Autodesk Inventor part; units mm, degrees
ref_plane "YZ Plane" through (0, 0, 0) normal (1, 0, 0) x (0, 1, 0)
ref_plane "XZ Plane" through (0, 0, 0) normal (0, 1, 0) x (-1, 0, 0)
ref_plane "XY Plane" through (0, 0, 0) normal (0, 0, 1) x (1, 0, 0)
sketch "Sketch8" plane through (0, 0, 0) normal (0, 1, 0) x (-1, 0, 0)
  line L0 (-13.5, -17.5) -> (13.5, -17.5)
  line L1 (13.5, -17.5) -> (13.5, 17.5)
  line L2 (13.5, 17.5) -> (-13.5, 17.5)
  line L3 (-13.5, 17.5) -> (-13.5, -17.5)
  line L4 (-13.5, -17.5) -> (13.5, 17.5) construction
  line L5 (13.5, -17.5) -> (-13.5, 17.5) construction
  circle A0 centre (10, -7.5) radius 1.6
  circle A1 centre (10, 7.5) radius 1.6
  circle A2 centre (-10, 7.5) radius 1.6
  circle A3 centre (-10, -7.5) radius 1.6
  point P0 (0, 0)
  dimension "d38" = 35
  dimension "d39" = 27
  dimension "d40" = 20
  dimension "d41" = 15
  dimension "d42" = 7.5
  dimension "d43" = 10
  dimension "d44" = 3.2
extrude "Extrusion7" add sketch "Sketch8" against normal blind 3
sketch "Sketch14" plane through (0, 0, 0) normal (0, 1, 0) x (1, 0, 0)
  line L0 (-13.5, 17.5) -> (-13.5, -17.5)
  line L1 (-13.5, -17.5) -> (13.5, -17.5)
  line L2 (13.5, -17.5) -> (13.5, 17.5)
  line L3 (13.5, 17.5) -> (-13.5, 17.5)
  circle A0 centre (-10, 7.5) radius 1.6
  circle A1 centre (-10, -7.5) radius 1.6
  circle A2 centre (10, -7.5) radius 1.6
  circle A3 centre (10, 7.5) radius 1.6
  line L4 (13.5, -17.5) -> (13.5, 17.5)
  line L5 (13.5, 4.5) -> (7.5, 4.5)
  line L6 (7.5, 4.5) -> (7.5, -4.5)
  line L7 (7.5, -4.5) -> (13.5, -4.5)
  line L8 (13.5, -4.5) -> (13.5, 4.5)
  point P0 (0, 0)
  dimension "d79" = 7.5
  dimension "d80" = 3
  dimension "d81" = 3
extrude "Extrusion12" add sketch "Sketch14" along normal blind 22.3 contours L2 L7 L6 L5
sketch "Sketch15" plane through (13.5, -3, 17.5) normal (1, 0, 0) x (0, 0, -1)
  line L0 (0, 3) -> (13, 3)
  line L1 (0, 3) -> (0, 0)
  line L2 (35, 0) -> (0, 0)
  line L3 (35, 3) -> (35, 0)
  line L4 (22, 3) -> (35, 3)
  line L5 (22, 3) -> (22, 25.3)
  line L6 (13, 25.3) -> (22, 25.3)
  line L7 (13, 3) -> (13, 25.3)
  line L8 (35, 3) -> (35, 0)
  line L9 (35, 0) -> (41.8017, 14.6399)
  circle A0 centre (35, 17.8) radius 2.6
  circle A1 centre (35, 17.8) radius 7.5
  circle A2 centre (0, 17.8) radius 2.6
  circle A3 centre (0, 17.8) radius 7.5
  line L10 (-275, -9) -> (225, -9)
  line L11 (0, 0) -> (-6.8017, 14.6399)
  line L12 (0, 25.3) -> (35, 25.3)
  point P0 (17.5, 3)
  point P1 (13, 25.3)
  point P2 (22, 25.3)
  dimension "d84" = 5.2
  dimension "d85" = 35
  dimension "d86" = 17.5
  dimension "d87" = 26.8
  dimension "d88" = 15
extrude "Extrusion13" add sketch "Sketch15" against normal blind 3 contours L1 L11 A3 L12 L7 L0 | L3 L4 L5 L12 A1 L9 | A3 | A1
sketch "Sketch16" plane through (10.5, -3, 17.5) normal (-1, 0, 0) x (0, 0, 1)
  arc A0 (-35, 25.3) -> (-41.8017, 14.6399) centre (-35, 17.8) ccw
  line L0 (-41.8017, 14.6399) -> (-35, 0)
  line L1 (-35, 3) -> (-35, 0)
  line L2 (-26.5199, 3) -> (-35, 3)
  line L3 (-26.5199, 3) -> (-23.4801, 3)
  line L4 (-22, 3) -> (-23.4801, 3)
  line L5 (-22, 25.3) -> (-22, 3)
  line L6 (-22, 25.3) -> (-35, 25.3)
  circle A1 centre (-35, 17.8) radius 2.6
  arc A2 (6.8017, 14.6399) -> (0, 25.3) centre (0, 17.8) ccw
  line L7 (0, 25.3) -> (-13, 25.3)
  line L8 (-13, 3) -> (-13, 25.3)
  line L9 (-11.5199, 3) -> (-13, 3)
  line L10 (-11.5199, 3) -> (-8.4801, 3)
  line L11 (0, 3) -> (-8.4801, 3)
  line L12 (0, 0) -> (0, 3)
  line L13 (0, 0) -> (6.8017, 14.6399)
  circle A3 centre (0, 17.8) radius 2.6
  line L14 (-22, 3) -> (-29, 3)
  line L15 (-29, 3) -> (-29, 13)
  line L16 (-29, 13) -> (-22, 13)
  line L17 (-22, 13) -> (-22, 3)
  line L18 (-11.5199, 3) -> (-13, 3)
  line L19 (-13, 3) -> (-6, 3)
  line L20 (-6, 3) -> (-6, 13)
  line L21 (-6, 13) -> (-13, 13)
  line L22 (-13, 13) -> (-13, 3)
  line L23 (-23.4, 0) -> (-26.6, 0)
  line L24 (-26.6, 3) -> (-23.4, 3)
  line L25 (-8.4, 0) -> (-11.6, 0)
  line L26 (-11.6, 3) -> (-8.4, 3)
  point P0 (-17.5, 3)
  point P1 (-10, 0)
  point P2 (-6, 3)
  dimension "d91" = 7
  dimension "d92" = 3
  dimension "d93" = 10
extrude "Extrusion14" cut sketch "Sketch16" against normal blind 22.3 contours L5 L4 L3 L2 L15 L16 | L21 L20 L11 L10 L9 L8
sketch "Sketch17" plane through (10.5, -3, 17.5) normal (-1, 0, 0) x (0, 0, 1)
  circle A0 centre (-35, 17.8) radius 2.6
  line L0 (-29, 3) -> (-29, 13)
  line L1 (-29, 13) -> (-22, 13)
  line L2 (-22, 25.3) -> (-22, 13)
  line L3 (-22, 25.3) -> (-35, 25.3)
  arc A1 (-35, 25.3) -> (-41.8017, 14.6399) centre (-35, 17.8) ccw
  line L4 (-41.8017, 14.6399) -> (-35, 0)
  line L5 (-35, 3) -> (-35, 0)
  line L6 (-29, 3) -> (-35, 3)
  circle A2 centre (0, 17.8) radius 2.6
  line L7 (-13, 13) -> (-6, 13)
  line L8 (-6, 13) -> (-6, 3)
  line L9 (0, 3) -> (-6, 3)
  line L10 (0, 0) -> (0, 3)
  line L11 (0, 0) -> (6.8017, 14.6399)
  arc A3 (6.8017, 14.6399) -> (0, 25.3) centre (0, 17.8) ccw
  line L12 (0, 25.3) -> (-13, 25.3)
  line L13 (-13, 13) -> (-13, 25.3)
  line L14 (-13, 13) -> (-10, 25.3)
  line L15 (-22, 13) -> (-25, 25.3)
  line L16 (-35, 25.3) -> (0, 25.3)
  point P0 (-17.5, 3)
  dimension "d96" = 15
extrude "Extrusion15" add sketch "Sketch17" along normal up to surface (3 mm away) contours L12 L14 L13 | L15 L3 L2
fillet "Fillet2" radius 2 2 edges at (9, 22.3, -7.5) (9, 22.3, 7.5)
mirror "Mirror1" about plane through (0, 0, 0) normal (1, 0, 0) of "Extrusion12", "Extrusion13", "Extrusion14", "Extrusion15", "Fillet2"
chamfer "Chamfer1" distance 5 angle 45 4 edges at (-10.5, 0, 14.5) (-10.5, 0, -14.5) (10.5, 0, 14.5) (10.5, 0, -14.5)
sketch "Sketch18" plane through (-13.5, 22.3, -17.5) normal (-1, 0, 0) x (0, 0, 1)
  line L0 (13, -22.3) -> (6, -22.3)
  line L1 (6, -22.3) -> (6, -12.3)
  line L2 (6, -12.3) -> (13, -12.3)
  line L3 (13, -12.3) -> (13, -22.3)
  line L4 (29, -22.3) -> (22, -22.3)
  line L5 (22, -22.3) -> (22, -12.3)
  line L6 (22, -12.3) -> (29, -12.3)
  line L7 (29, -12.3) -> (29, -22.3)
  circle A0 centre (0, -7.5) radius 2.6
  circle A1 centre (35, -7.5) radius 2.6
  line L8 (41.8017, -10.6601) -> (35, -25.3)
  arc A2 (41.8017, -10.6601) -> (35, 0) centre (35, -7.5) ccw
  line L9 (0, 0) -> (35, 0)
  arc A3 (0, 0) -> (-6.8017, -10.6601) centre (0, -7.5) ccw
  line L10 (0, -25.3) -> (-6.8017, -10.6601)
  line L11 (35, -25.3) -> (0, -25.3)
  point P0 (17.5, -22.3)
  point P1 (17.5, -7)
  point P2 (17.5, -15.3)
  dimension "d103" = 7
  dimension "d104" = 10
hole "Hole3" at (-13.5, 15.3, 0) at (-13.5, 7, 0) direction (1, 0, 0) diameter 3.6 end through all
sketch "Sketch19" plane through (13.5, 22.3, 17.5) normal (1, 0, 0) x (0, 0, -1)
  circle A0 centre (17.5, -15.3) radius 1.8
  circle A1 centre (17.5, -7) radius 1.8
  circle A2 centre (17.5, -15.3) radius 3.25
  circle A3 centre (17.5, -7) radius 3.25
  point P0 (17.5, -22.3)
  dimension "d112" = 6.5
extrude "Extrusion16" cut sketch "Sketch19" against normal blind 3 contours A0 | A1 | A2 | A3
sketch "Sketch20" plane through (-13.5, 22.3, -17.5) normal (-1, 0, 0) x (0, 0, 1)
  circle A0 centre (17.5, -15.3) radius 3.25
  circle A1 centre (17.5, -7) radius 3.25
  point P0 (17.5, -22.3)
extrude "Extrusion17" cut sketch "Sketch20" against normal blind 3
sketch "Sketch21" plane through (13.5, 22.3, 17.5) normal (1, 0, 0) x (0, 0, -1)
  circle A0 centre (17.5, -7) radius 3.25
  circle A1 centre (17.5, -15.3) radius 3.25
  line L0 (29, -22.3) -> (22, -22.3)
  line L1 (22, -22.3) -> (22, -12.3)
  line L2 (22, -12.3) -> (29, -12.3)
  line L3 (29, -12.3) -> (29, -22.3)
  line L4 (13, -22.3) -> (6, -22.3)
  line L5 (6, -22.3) -> (6, -12.3)
  line L6 (6, -12.3) -> (13, -12.3)
  line L7 (13, -12.3) -> (13, -22.3)
  circle A2 centre (0, -7.5) radius 2.6
  circle A3 centre (35, -7.5) radius 2.6
  line L8 (35, -25.3) -> (0, -25.3)
  line L9 (35, -25.3) -> (41.8017, -10.6601)
  arc A4 (41.8017, -10.6601) -> (35, 0) centre (35, -7.5) ccw
  line L10 (35, 0) -> (0, 0)
  arc A5 (0, 0) -> (-6.8017, -10.6601) centre (0, -7.5) ccw
  line L11 (-6.8017, -10.6601) -> (0, -25.3)
  arc A6 (41.8017, -10.6601) -> (35, 0) centre (35, -7.5) ccw
  line L12 (42.5, -7.5) -> (42.5, 0)
  line L13 (42.5, 0) -> (35, 0)
  line L14 (22.4536, 0) -> (35, 0)
  point P0 (17.5, -22.3)
extrude "Extrusion18" add sketch "Sketch21" against normal up to surface (3 mm away) contours A4 L13 L12
equation "\"d81\" = d80"
properties part number "Y Axis Gantry Baseblock (CNC)" material "ABS Plastic"
Verification items for the finished model (mm, model axes). A direction names the side the tool comes from. Coordinates: 2 decimals unless noted, no trailing zeros. Order: outer loops, then holes, each group sorted by start corner. A loop starts at its lowest first (then second) coordinate and runs counter-clockwise, first axis right, second up. Notation, with made-up numbers: M 19,-30.75 L 75,-30.75 A21 cw 75,-10.75 Z; hole C 29,11 d10. An arc over 180 degrees is marked long. One line per item, written item: value. Start each with the question number.
Item 1: Sectioned sample at A-A (z = 7.5). Enter the section's corners in (x, y).
Item 2: Scan lines: probe 1 along X at (y, z) = (-1.65, 7.5); probe 2 along Y at (x, z) = (-9, 0); probe 3 along Y at (x, z) = (12.9, 0). Record each from-to range of solid material in increasing order.
Item 3: Sectioned sample at C-C (x = -6.5). Enter the section's corners in (y, z).
Item 4: Mould release check, pull along Z, two halves, no side actions. Record for faces 4 (the flat face through (10, 5, 4.5)), 5 (the flat face through (11, 22.3, -4)), 6 (the cylindrical face through (9.021, 13.515, -0.234)), 7 (the cylindrical face through (8.979, 21.555, -6.511)): released by +Z, released by -Z, zero draft, split by the parting line, or undercut.
Item 5: Gauge pin test, flat ends, axial feed: pin 1 (4 mm diameter, centred on y = 15.3, z = 0, fed in from +X); pin 2 (12 mm diameter, centred on x = -7.5, z = 19, fed in from +Y); pin 3 (6.5 mm diameter, centred on x = -11, y = 7, fed in from +Z); pin 4 (3 mm diameter, centred on x = 10.5, y = 0.5, fed in from +Z). Record the tip position at first contact, or that the pin passes through.
Item 6: Sectioned sample at B-B (y = 20.5). Enter the section's corners in (x, z).
Item 7: Access from +Z, -Z, +X, -X, +Y, -Y to the whole of each face (thin tool, end or side, straight path). Record for faces 1 (the flat face through (-10.5, 5.6, 1.4)), 2 (the cylindrical face through (-8.73, -1.48, 6.53)), 3 (the cylindrical face through (12.021, 10.222, 0.423)).
Item 8: Sectioned sample at D-D (z = 13.5). Enter the section's corners in (x, y).
Conclusion:
1. outline: M -13.5,-3 L -11.6,-3 L -11.6,0 L -13.5,0 Z; M -13.5,10 L -10.5,10 L -10.5,22.3 L -13.5,22.3 Z; M -8.4,-3 L 8.4,-3 L 8.4,0 L -8.4,0 Z; M 10.5,10 L 13.5,10 L 13.5,22.3 L 10.5,22.3 Z; M 11.6,-3 L 13.5,-3 L 13.5,0 L 11.6,0 Z
2. probe 1: x = -13.5 to -11.6, -8.4 to 8.4, 11.6 to 13.5
2. probe 2: y = -3 to 5.2, 8.8 to 13.5, 17.1 to 22.3
2. probe 3: y = -3 to 3.75, 10.25 to 12.05, 18.55 to 22.3
3. outline: M -3,-17.5 L 1,-17.5 L 1,-11.5 L 0,-11.5 L 0,11.5 L 1,11.5 L 1,17.5 L -3,17.5 Z
4. face 4: undercut
4. face 5: zero draft
4. face 6: undercut
4. face 7: released by -Z
5. pin 1: stops at x = 10.5
5. pin 2: stops at y = 22.3
5. pin 3: stops at z = 23.66
5. pin 4: stops at z = 19.82
6. outline: M -13.5,-22.37 L -10.5,-22.37 L -10.5,-6.94 L -7.5,-6.94 L -7.5,6.94 L -10.5,6.94 L -10.5,22.37 L -13.5,22.37 Z; M 7.5,-6.94 L 10.5,-6.94 L 10.5,-25 L 13.5,-25 L 13.5,22.37 L 10.5,22.37 L 10.5,6.94 L 7.5,6.94 Z
7. face 1: -X
7. face 2: -Y
7. face 3: +X
8. outline: M -13.5,-3 L 13.5,-3 L 13.5,22.3 L 10.5,22.3 L 10.5,5 L 5.5,0 L -5.5,0 L -10.5,5 L -10.5,22.3 L -13.5,22.3 Z
